Autodesk Inventor part; units mm, degrees
ref_plane "YZ Plane" through (0, 0, 0) normal (1, 0, 0) x (0, 1, 0)
ref_plane "XZ Plane" through (0, 0, 0) normal (0, 1, 0) x (-1, 0, 0)
ref_plane "XY Plane" through (0, 0, 0) normal (0, 0, 1) x (1, 0, 0)
sketch "Sketch1" plane through (0, 0, 0) normal (0, 0, 1) x (1, 0, 0)
  circle A0 centre (0, 0) radius 7.3825
  dimension "d0" = 14.765
extrude "Extrusion1" add sketch "Sketch1" along normal mid plane 55.56
sketch "Sketch3" plane through (0, 0, 27.78) normal (0, 0, 1) x (1, 0, 0)
  circle A0 centre (0, 0) radius 3.5725
  dimension "d6" = 7.145
extrude "Extrusion2" cut sketch "Sketch3" against normal blind 16.6675
sketch "Sketch4" plane through (0, 0, 0) normal (1, 0, 0) x (0, 1, 0)
  circle A0 centre (0, -23.4163) radius 0.9525
  point P0 (0, 0)
  dimension "d9" = 23.4163
  dimension "d10" = 1.905
extrude "Extrusion3" cut sketch "Sketch4" along normal through all both and the other way through all
sketch "Sketch6" plane through (0, 0, 0) normal (1, 0, 0) x (0, 1, 0)
  line L0 (-3.5725, 27.78) -> (3.5725, 27.78)
  line L1 (-3.5725, 11.1125) -> (3.5725, 11.1125)
  line L2 (3.5725, 27.78) -> (3.0645, 27.78)
  line L3 (3.0645, 27.78) -> (3.0645, 11.1125)
  line L4 (3.0645, 11.1125) -> (3.5725, 11.1125)
  line L5 (3.5725, 11.1125) -> (3.5725, 27.78)
  point P0 (0, 0)
  dimension "d17" = 0.508
extrude "Extrusion5" add sketch "Sketch6" along normal mid plane 0.8636
mirror "Mirror5" about plane through (0, 0, 0) normal (0, 0, 1) of "Extrusion5", "Extrusion3", "Extrusion2"
properties part number "Wheel_axis_3DPrint"
Geometry: final body of the model. Coordinates: model frame, mm. Give positions to 0.01 mm unless a question says otherwise; leave off trailing zeros. Write each loop counter-clockwise with the first axis right and the second up, starting at its lowest first coordinate (ties: lowest second). Pieces come first, ordered by that corner, then holes. Notation, with made-up numbers: (-10.5, 33.25) - (38.5, 33.25) arc R19 cw to (38.5, 39.25) - close; hole circle Ø6 at (21, -25). An arc over 180 degrees is marked (long way). Return JSON: item names as keys, results as strings. Group by question number.
1) Section C-C on x = 1. Return the cut outline in (y, z), plus the area to 3 significant figures.
2) Section B-B on z = 18. Return the cut outline in (x, y) (1 decimal), plus the area to 3 significant figures.
3) Line query: line 1 (Z direction, x = 5.6, y = 0); line 2 (X direction, y = 0, z = -17); line 3 (X direction, y = -0.25, z = 10.5). Output: solid intervals per line, ascending.
4) Section D-D on y = 2.5. Return the cut outline in (x, z).
5) Section A-A on y = 0. Return the cut outline in (x, z), plus the area to 3 significant figures.
6) First-contact query: P1, Ø5, axis at y = 0.5, z = 10.5, coming from the +X side; P2, Ø2, axis at x = -1.5, y = -0.5, coming from the +Z side; P3, Ø1.5, axis at y = -5.5, z = 19.5, coming from the -X side; P4, Ø1, axis at y = -5, z = 7, coming from the +X side. Flat tips, straight axial feed; report the tip coordinate or a pass-through.
7) Mould query, pull axis X, two halves, no side actions, for faces 1 (the cylindrical face through (-5.385, -0.206, 22.486)), 2 (the flat face through (0, 0, -11.112)), 3 (the cylindrical face through (7.04, -2.22, -0.39)), 4 (the cylindrical face through (0.15, -3.57, -19.56)). Classes: released by +X, released by -X, zero draft, split by the parting line, or undercut.
Filled in:
{
 "1": {"outline": "(-7.31, -27.78) - (-3.43, -27.78) - (-3.43, -11.11) - (3.43, -11.11) - (3.43, -27.78) - (7.31, -27.78) - (7.31, 27.78) - (3.43, 27.78) - (3.43, 11.11) - (-3.43, 11.11) - (-3.43, 27.78) - (-7.31, 27.78) - close", "area": "584 mm^2"},
 "2": {"outline": "circle Ø14.8 at (0, 0); hole (-0.4, 3.1) - (-0.4, 3.5) arc R3.6 ccw (long way) to (0.4, 3.5) - (0.4, 3.1) - close", "area": "132 mm^2"},
 "3": {"line 1": "z = -27.78 to -24.37, -22.46 to 22.46, 24.37 to 27.78", "line 2": "x = -7.38 to -3.57, 3.57 to 7.38", "line 3": "x = -7.38 to 7.38"},
 "4": {"outline": "(-6.95, -27.78) - (-2.55, -27.78) - (-2.55, -11.11) - (2.55, -11.11) - (2.55, -27.78) - (6.95, -27.78) - (6.95, 27.78) - (2.55, 27.78) - (2.55, 11.11) - (-2.55, 11.11) - (-2.55, 27.78) - (-6.95, 27.78) - close"},
 "5": {"outline": "(-7.38, -27.78) - (-3.57, -27.78) - (-3.57, -24.37) - (-7.38, -24.37) - close; (-7.38, -22.46) - (-3.57, -22.46) - (-3.57, -11.11) - (3.57, -11.11) - (3.57, -22.46) - (7.38, -22.46) - (7.38, 22.46) - (3.57, 22.46) - (3.57, 11.11) - (-3.57, 11.11) - (-3.57, 22.46) - (-7.38, 22.46) - close; (-7.38, 24.37) - (-3.57, 24.37) - (-3.57, 27.78) - (-7.38, 27.78) - close; (3.57, -27.78) - (7.38, -27.78) - (7.38, -24.37) - (3.57, -24.37) - close; (3.57, 24.37) - (7.38, 24.37) - (7.38, 27.78) - (3.57, 27.78) - close", "area": "553 mm^2"},
 "6": {"P1": "stops at x = 7.38", "P2": "stops at z = 11.11", "P3": "stops at x = -5.65", "P4": "stops at x = 5.85"},
 "7": {"face 1": "zero draft", "face 2": "undercut", "face 3": "split by the parting line", "face 4": "undercut"}
}
